Autodesk Inventor part; units mm, degrees
ref_plane "YZ Plane" through (0, 0, 0) normal (1, 0, 0) x (0, 1, 0)
ref_plane "XZ Plane" through (0, 0, 0) normal (0, 1, 0) x (-1, 0, 0)
ref_plane "XY Plane" through (0, 0, 0) normal (0, 0, 1) x (1, 0, 0)
sketch "Skizze1" plane through (0, 0, 0) normal (0, 0, 1) x (1, 0, 0)
  line L0 (-30, -80) -> (30, -80)
  line L1 (30, -80) -> (30, 80)
  line L2 (30, 80) -> (-30, 80)
  line L3 (-30, 80) -> (-30, -80)
  line L4 (-30, -80) -> (30, 80) construction
  line L5 (30, -80) -> (-30, 80) construction
  point P0 (0, 0)
  dimension "d0" = 60
  dimension "d1" = 160
extrude "Extrusion1" add sketch "Skizze1" along normal blind 100
sketch "Skizze5" plane through (30, -80, 0) normal (1, 0, 0) x (0, 0, -1)
  line L0 (0, 0) -> (-70, 0)
  line L1 (-70, 0) -> (-70, 13)
  line L2 (-70, 13) -> (0, 13)
  line L3 (0, 13) -> (0, 0)
  point P0 (0, 80)
  dimension "d15" = 70
  dimension "d16" = 13
extrude "Extrusion5" cut sketch "Skizze5" against normal through all
sketch "Skizze6" plane through (30, 80, 100) normal (1, 0, 0) x (0, 0, -1)
  line L0 (100, 0) -> (0, 0)
  line L1 (0, 0) -> (30, 0)
  line L2 (30, 0) -> (30, 12)
  line L3 (30, 12) -> (0, 12)
  line L4 (0, 12) -> (0, 0)
  point P0 (100, -80)
  point P1 (30, 0)
  dimension "d24" = 30
  dimension "d25" = 12
extrude "Extrusion6" add sketch "Skizze6" against normal up to surface (60 mm away)
fillet "Rundung1" radius 10 2 edges at (0, -67, 0) (0, 80, 0)
sketch "Skizze7" plane through (30, -80, 70) normal (1, 0, 0) x (0, 0, -1)
  line L0 (-30, 0) -> (-17.65, 0)
  line L1 (0, 0) -> (-30, 0)
  line L2 (-30, 0) -> (-30, 172)
  line L3 (-30, 0) -> (-30, 172)
  spline S0 degree 2 poles (-30, 172) (-30, 85.6679) (-17.65, 0) knots 0 0 0 1 1 1
  point P0 (70, 80)
  dimension "d27" = 12.35
extrude "Extrusion7" cut sketch "Skizze7" against normal up to next
equation "\"G_L\" = 0"
equation "\"G_H\" = 0"
equation "\"G_B\" = 0"
properties part number "canopy" material "PC/ABS-Kunststoff"
The model under review builds one solid part; all positions refer to its coordinate system, in mm. A direction names the side the tool comes from. Give positions to 0.01 mm unless a question says otherwise; leave off trailing zeros. Order: outer loops, then holes, each group sorted by start corner. A loop starts at its lowest first (then second) coordinate and runs counter-clockwise, first axis right, second up. Notation, with made-up numbers: (79.5, -6) -> (109.5, -6) arc R11 ccw to (109.5, 15) -> close; hole circle Ø5 at (-27.75, 62). An arc over 180 degrees is marked (long way). Write item = value, one per line. Start each with the question number.
(1) Tool access review of faces 1 (the flat face through (0, -80, 79)), 2 (the flat face through (0, -67, 40)), 3 (the flat face through (0, 80, 40)): name each direction out of +Z, -Z, +X, -X, +Y, -Y from which nothing blocks a thin tool from reaching the whole face with its end or side.
(2) For L1, parallel to Y at x = -22.5, z = 50; L2, parallel to Z at x = 23.5, y = 51; L3, parallel to Z at x = -5.5, y = 22.5, list the stretches that pass through material, from the lowest coordinate up. Write a range as from..to.
(3) For pin 1 Ø14.5 at (x, y) = (14.5, -71) entering from -Z; pin 2 Ø12 at (x, y) = (-2.5, 40) entering from -Z; pin 3 Ø1 at (x, y) = (2, -2.5) entering from +Z; pin 4 Ø6 at (x, y) = (6.5, 88) entering from -Z, all flat-tipped, find the tip position at first contact; note any pin that passes through.
(4) Take a section at A-A (z = 22.5). Write out the cut boundary in (x, y).
Returned:
q1.face_1 = +Z, -Z, +X, -X, -Y
q1.face_2 = -Z, +X, -X, -Y
q1.face_3 = -Z, +X, -X, +Y
q2.L1 = -67..80
q2.L2 = 0..99.3
q2.L3 = 0..97.99
q3.pin_1 = 2.62
q3.pin_2 = 0
q3.pin_3 = 96.32
q3.pin_4 = 70
q4.outline = (-30, -67) -> (30, -67) -> (30, 80) -> (-30, 80) -> close
